The listing builds one solid part. Answer for the finished solid, in the listing's coordinates (mm). A direction names the side the tool comes from. Coordinates: 2 decimals unless noted, no trailing zeros. Loops run counter-clockwise (first coordinate to the right, second up) from the corner with the lowest first, then second, coordinate; pieces in that order, holes last. Notation, with made-up numbers: (52, 26) - (75, 26) arc R17 ccw to (75, 30) - close; hole circle Ø10 at (-16, 79). An arc over 180 degrees is marked (long way). Return JSON: item names as keys, results as strings. Group by question number.
1. Section D-D (z = 4.75) is taken. Write down the section's boundary in (x, y), and give its area (3 significant figures).
2. Section B-B (x = 12.8) is taken. Write down the section's boundary in (y, z).
3. Which of the six approach directions +Z, -Z, +X, -X, +Y, -Y give full straight-line access (tool end or side, diameter ignored) to faces 1 (the face through (23, 14, 9)), 2 (the face through (6, 26, 11)), 3 (the face through (-30, 6, 5.7)), 4 (the face through (32, 6, 5.7)), 5 (the face through (35.4, 2.96, 14.43))?
4. Find the intervals of material crossed by line 1 along X through (y, z) = (3.2, 7.5); line 2 along Z through (x, y) = (-31, 4.25); line 3 along Y through (x, z) = (-7, 8.5), in increasing order.
5. Each of these flat-tipped pins is pushed along its axis until it touches: P1, Ø3, axis at y = 27, z = 10, coming from the +X side; P2, Ø1.8, axis at x = -2.5, y = 26, coming from the +Z side; P3, Ø3, axis at x = 31.5, z = 11, coming from the +Y side; P4, Ø2, axis at x = 31, z = 7.5, coming from the +Y side. Where does it stop, or does it pass through?
6. Section A-A (z = 10.5) is taken. Write down the section's boundary in (x, y), and give its area (3 significant figures).
7. The mould has two halves that part along Z. Classify faces 6 (the face through (0, 14, 3)), 7 (the face through (29.43, 2.96, 8.15)), 8 (the face through (-26, 16, 7)): pulls with the +Z half, pulls with the -Z half, needs draft (parallel to the pull), parting line crosses it, or undercut.
8. Section C-C (y = 14) is taken. Write down the section's boundary in (x, z), and give its area (3 significant figures).
```python
from build123d import *

# Parameters (mm, degrees)
BOSS_EXTRU_1_DEPTH      = 15
ESQUISSE2_W             = 46
ESQUISSE2_H             = 21
ENL_V_MAT_EXTRU_1_DEPTH = 12
ESQUISSE4_R             = 8
ENL_V_MAT_EXTRU_2_DEPTH = 3
ENL_V_MAT_EXTRU_3_REACH = 50.01
ESQUISSE5_W             = 12
ESQUISSE5_H             = 7
CONG_1_R                = 2
D_GAGEMENT_M31_D        = 3.4


with BuildPart() as part:
    # Esquisse1 → Boss.-Extru.1 (new body)
    with BuildSketch(Plane.XY):
        Polygon((36, 0), (-36, 0), (-36, 6), (-26, 6), (-26, 28), (26, 28), (26, 6), (36, 6), align=None)
    extrude(amount=BOSS_EXTRU_1_DEPTH)

    # Esquisse2 → Enlèv. mat.-Extru.1 (cut)
    with BuildSketch(Plane.XY.offset(15)):
        with Locations((0, 14)):
            Rectangle(ESQUISSE2_W, ESQUISSE2_H)
    extrude(amount=-ENL_V_MAT_EXTRU_1_DEPTH, mode=Mode.SUBTRACT)

    # Esquisse4 → Enlèv. mat.-Extru.2 (cut)
    with BuildSketch(Plane.XY.offset(3)):
        with Locations((-12.8, 14)):
            Circle(ESQUISSE4_R)
        with Locations((12.8, 14)):
            Circle(ESQUISSE4_R)
    extrude(amount=-ENL_V_MAT_EXTRU_2_DEPTH, mode=Mode.SUBTRACT)

    # Enlèv. mat.-Extru.3: up to this face of the body (flat: up to its plane)
    enl_v_mat_extru_3_end = Plane(part.part.faces().sort_by_distance((0, 28, 7.5))[0])
    # Esquisse5 → Enlèv. mat.-Extru.3 (cut, up to the picked face)
    with BuildSketch(Plane.XZ, mode=Mode.PRIVATE) as enl_v_mat_extru_3_sk1:
        with Locations((0, 11.5)):
            Rectangle(ESQUISSE5_W, ESQUISSE5_H)
    enl_v_mat_extru_3_tool1 = split(extrude(enl_v_mat_extru_3_sk1.sketch, amount=-ENL_V_MAT_EXTRU_3_REACH, mode=Mode.PRIVATE), bisect_by=enl_v_mat_extru_3_end, keep=Keep.BOTH, mode=Mode.PRIVATE)
    add(enl_v_mat_extru_3_tool1.solids().sort_by(Axis((0, 0, 11.5), (0, 1, 0)))[0], mode=Mode.SUBTRACT)

    # Congé1
    cong_1_edges = [part.edges().sort_by_distance(p)[0] for p in [
        (36, 3, 0),
        (-36, 3, 0),
        (36, 3, 15),
        (-26, 28, 7.5),
        (26, 28, 7.5),
        (-36, 3, 15),
    ]]
    fillet(cong_1_edges, radius=CONG_1_R)

    # Dégagement M31 (through all)
    with Locations(Plane(origin=(0, 6, 0), x_dir=(1, 0, 0), z_dir=(0, 1, 0))):
        with Locations((-31, -7.5), (31, -7.5)):
            Hole(D_GAGEMENT_M31_D / 2)


solid = part.part
```
The answers:
{
 "1": {"outline": "(-36, 0) - (36, 0) - (36, 6) - (26, 6) - (26, 26) arc R2 ccw to (24, 28) - (-24, 28) arc R2 ccw to (-26, 26) - (-26, 6) - (-36, 6) - close; hole (-23, 3.5) - (23, 3.5) - (23, 24.5) - (-23, 24.5) - close", "area": "608 mm2"},
 "2": {"outline": "(0, 0) - (6, 0) - (6, 3) - (3.5, 3) - (3.5, 15) - (0, 15) - close; (22, 0) - (28, 0) - (28, 15) - (24.5, 15) - (24.5, 3) - (22, 3) - close"},
 "3": {"face 1": "+Z", "face 2": "+Z, +Y, -Y", "face 3": "+Z, -Z, -X, +Y", "face 4": "+Z, -Z, +X, +Y", "face 5": "+Z, +X, +Y, -Y"},
 "4": {"line 1": "x = -36 to -32.7, -29.3 to 29.3, 32.7 to 36", "line 2": "z = 0 to 5.8, 9.2 to 15", "line 3": "y = 0 to 3.5, 24.5 to 28"},
 "5": {"P1": "stops at x = 26", "P2": "stops at z = 8", "P3": "stops at y = 6", "P4": "passes through"},
 "6": {"outline": "(-36, 0) - (-6, 0) - (-6, 3.5) - (-23, 3.5) - (-23, 24.5) - (-6, 24.5) - (-6, 28) - (-24, 28) arc R2 ccw to (-26, 26) - (-26, 6) - (-36, 6) - close; (6, 0) - (36, 0) - (36, 6) - (26, 6) - (26, 26) arc R2 ccw to (24, 28) - (6, 28) - (6, 24.5) - (23, 24.5) - (23, 3.5) - (6, 3.5) - close", "area": "524 mm2"},
 "7": {"face 6": "pulls with the +Z half", "face 7": "undercut", "face 8": "needs draft"},
 "8": {"outline": "(-26, 0) - (-20.8, 0) - (-20.8, 3) - (-23, 3) - (-23, 15) - (-26, 15) - close; (-4.8, 0) - (4.8, 0) - (4.8, 3) - (-4.8, 3) - close; (20.8, 0) - (26, 0) - (26, 15) - (23, 15) - (23, 3) - (20.8, 3) - close", "area": "132 mm2"}
}
